The model under review builds one solid part; all positions refer to its coordinate system, in mm. A direction names the side the tool comes from. Coordinates: 2 decimals unless noted, no trailing zeros. Loops run counter-clockwise (first coordinate to the right, second up) from the corner with the lowest first, then second, coordinate; pieces in that order, holes last. Notation, with made-up numbers: (59.5, 77) - (95.5, 77) arc R12 cw to (95.5, 95) - close; hole circle Ø11 at (-19.5, 45). An arc over 180 degrees is marked (long way). One line per item, written item: value. Start each with the question number.
1. Insertion check: P1, Ø3, axis at x = -6.5, z = 50.5, coming from the +Y side; P2, Ø8, axis at y = 1.5, z = 58, coming from the +X side; P3, Ø12, axis at x = 0, z = 64, coming from the -Y side. Each pin has a flat end and moves straight along its axis. Give the tip position at first contact, or say it passes through.
2. For faces 1 (the face through (15, 0, -1)), 2 (the face through (12, 0, 58)), 3 (the face through (0, -5, 58)), 4 (the face through (-12, 0, 58)), 5 (the face through (0, 5, 58)), list the 3-axis set-ups (+Z, -Z, +X, -X, +Y, -Y) from which the entire face can be reached by the end or side of a thin tool; tool diameter is ignored.
3. To check wall thickness, follow line 1 (Z direction, x = -6.25, y = 5.5); line 2 (Y direction, x = 5, z = 59). State the ranges of each line that lie inside material, in increasing order.
4. We need section B-B, the plane x = -6. Give the boundary of the cut face in (y, z), then the cut area to 3 significant figures.
5. We need section A-A, the plane y = 3.5. Give the boundary of the cut face in (x, z).
from build123d import *

# Parameters (mm, degrees)
F1_DEPTH = 10
F2_DEPTH = 10
F0_W     = 24
F0_H     = 24
F3_DEPTH = 5
F4_DEPTH = 5


with BuildPart() as f1:
    # F0 (on Front) → F1 (new body)
    with BuildSketch(Plane.XZ):
        Polygon((15, 46.178577), (12, 46.178577), (-12, 46.178577), (-15, 46.178577), (-15, -20.821423), (-15, -46.178577), (0, -46.178577), (15, -46.178577), (15, -20.821423), align=None)
    extrude(amount=F1_DEPTH)

    # F0 (on Front) → F2 (join)
    with BuildSketch(Plane.XZ):
        Polygon((15, 46.178577), (12, 46.178577), (-12, 46.178577), (-15, 46.178577), (-15, -20.821423), (-15, -46.178577), (0, -46.178577), (15, -46.178577), (15, -20.821423), align=None)
    extrude(amount=-F2_DEPTH)

    # F0 (on Front) → F3 (join)
    with BuildSketch(Plane.XZ):
        with Locations((0, 58.178577)):
            Rectangle(F0_W, F0_H)
    extrude(amount=-F3_DEPTH)

    # F0 (on Front) → F4 (join)
    with BuildSketch(Plane.XZ):
        with Locations((0, 58.178577)):
            Rectangle(F0_W, F0_H)
    extrude(amount=F4_DEPTH)


solid = f1.part
Findings below:
1. P1: y = 5
1. P2: x = 12
1. P3: y = -5
2. face 1: +Z, -Z, +X, +Y, -Y
2. face 2: +Z, +X, +Y, -Y
2. face 3: +Z, +X, -X, -Y
2. face 4: +Z, -X, +Y, -Y
2. face 5: +Z, +X, -X, +Y
3. line 1: -46.18 to 46.18
3. line 2: -5 to 5
4. outline: (-10, -46.18) - (10, -46.18) - (10, 46.18) - (5, 46.18) - (5, 70.18) - (-5, 70.18) - (-5, 46.18) - (-10, 46.18) - close
4. area: 2,090 mm2
5. outline: (-15, -46.18) - (15, -46.18) - (15, 46.18) - (12, 46.18) - (12, 70.18) - (-12, 70.18) - (-12, 46.18) - (-15, 46.18) - close
